```python
from build123d import *

# Parameters (mm, degrees)
SKIZZE1_R                       = 2
AUFSATZ_LINEAR_AUSTRAGEN1_DEPTH = 67.5
SKIZZE7_W                       = 0.5
SKIZZE7_H                       = 0.1
SCHNITT_LINEAR_AUSTRAGEN1_DEPTH = 27
FASE1_SIZE                      = 0.2


with BuildPart() as part:
    # Skizze1 → Aufsatz-Linear austragen1 (new, symmetric)
    with BuildSketch(Plane.XY):
        Circle(SKIZZE1_R)
    extrude(amount=AUFSATZ_LINEAR_AUSTRAGEN1_DEPTH, both=True)

    # Skizze7 → Schnitt-Rotation1 (revolve, cut)
    with BuildSketch(Plane(origin=(0, 0, 0), x_dir=(0, 0, -1), z_dir=(1, 0, 0))):
        with Locations((-66.75, 1.95)):
            Rectangle(SKIZZE7_W, SKIZZE7_H)
        with Locations((54.25, 1.95)):
            Rectangle(SKIZZE7_W, SKIZZE7_H)
    revolve(axis=Axis((0, 0, -67.5), (0, 0, 1)), mode=Mode.SUBTRACT)

    # Skizze8 → Schnitt-Linear austragen1 (cut)
    with BuildSketch(Plane.XY.offset(67.5)):
        with BuildLine():
            Line((1.2, 1.6), (-1.2, 1.6))
            ThreePointArc((-1.2, 1.6), (0, 2), (1.2, 1.6))
        make_face()
    extrude(amount=-SCHNITT_LINEAR_AUSTRAGEN1_DEPTH, mode=Mode.SUBTRACT)

    # Fase1
    fase1_edges = [part.edges().sort_by_distance(p)[0] for p in [
        (-2, 0, -67.5),
        (0, -2, 67.5),
    ]]
    chamfer(fase1_edges, length=FASE1_SIZE)


solid = part.part
```
Source: CAD feature listing. Evaluate the final solid. Frame: model axes, mm. A direction names the side the tool comes from. Coordinates: 2 decimals unless noted, no trailing zeros. Loops run counter-clockwise (first coordinate to the right, second up) from the corner with the lowest first, then second, coordinate; pieces in that order, holes last. Notation, with made-up numbers: M -21,54 L 15,54 A23 ccw 15,89 Z; hole C 25.25,18 d9. An arc over 180 degrees is marked long. Use a Markdown table: item, result. Add a question column.
Q1. Access query for faces 1 (the cylindrical face through (-0.08, -1.9, -54.25)), 2 (the flat face through (0, 1.6, 54)), 3 (the cylindrical face through (0, -2, 7)). Directions: +Z, -Z, +X, -X, +Y, -Y. A direction counts if a zero-diameter tool reaches every point of the face in a straight line with its end or side. Return the directions, or none.
Q2. Material intervals for L1, parallel to Y at x = 0.65, z = 44.5; L2, parallel to X at y = -0.6, z = -8.5; L3, parallel to X at y = -1.6, z = 42.5, sorted ascending.
Q3. Section query B-B, the plane z = -45. Return loops of the section in (x, y), and give its area (3 significant figures).
Q4. Draft query along Z for faces 4 (the flat face through (0, 0, -67.5)), 5 (the cylindrical face through (-0.07, -2, 67.15)), 6 (the cylindrical face through (-0.07, -1.9, 66.75)). Return one class per face: pulls with the +Z half, pulls with the -Z half, needs draft (parallel to the pull), parting line crosses it, or undercut.
Q5. Section query A-A, the plane z = 51. Return loops of the section in (x, y).
Result:
| question | item | result |
|---|---|---|
| 1 | face 1 | none |
| 1 | face 2 | +Z, +X, -X, +Y |
| 1 | face 3 | +Z, -Z |
| 2 | L1 | y = -1.89 to 1.6 |
| 2 | L2 | x = -1.91 to 1.91 |
| 2 | L3 | x = -1.2 to 1.2 |
| 3 | outline | C 0,0 d4 |
| 3 | area | 12.6 mm2 |
| 4 | face 4 | pulls with the -Z half |
| 4 | face 5 | needs draft |
| 4 | face 6 | undercut |
| 5 | outline | M -1.2,1.6 A2 ccw long 1.2,1.6 Z |
